Read the model definition and answer for the solid it produces. Units are mm, in the model's axes. A direction names the side the tool comes from. Give positions to 0.01 mm unless a question says otherwise; leave off trailing zeros. Write each loop counter-clockwise with the first axis right and the second up, starting at its lowest first coordinate (ties: lowest second). Pieces come first, ordered by that corner, then holes. Notation, with made-up numbers: M -18,-16 L 24,-16 A19 cw 24,1 Z; hole C 87.5,16.25 d7. An arc over 180 degrees is marked long. Put each result on its own line as item: value.
from build123d import *

# Parameters (mm, degrees)
SKETCH1_R                 = 4.7625
SKETCH1_W                 = 6.5278
SKETCH1_H                 = 6.5278
SKETCH1_H_2               = 6.348837221
BOSS_EXTRUDE1_DEPTH       = 6.35
F_6_CLEARANCE_HOLE1_D     = 3.7973
F_6_CLEARANCE_HOLE1_DEPTH = 12.7
F_6_CLEARANCE_HOLE1_TIP   = 1.140824014
SKETCH7_W                 = 6.35
SKETCH7_H                 = 6.1722
BOSS_EXTRUDE2_DEPTH       = 1.016
SKETCH8_W                 = 6.35
SKETCH8_H                 = 6.1722
BOSS_EXTRUDE3_DEPTH       = 1.016
SKETCH9_R                 = 1.5875
CUT_EXTRUDE1_DEPTH        = 161.894515133


with BuildPart() as part:
    # Sketch1 → Boss-Extrude1 (new body)
    with BuildSketch(Plane(origin=(0, 0, 0), x_dir=(0, 0, -1), z_dir=(1, 0, 0))):
        Polygon((0, 0), (-14.664696837, 25.4), (-144.085303163, 25.4), (-158.75, 0), align=None)
        with Locations((-130.048, 12.7)):
            Circle(SKETCH1_R, mode=Mode.SUBTRACT)
        with Locations((-28.702, 12.7)):
            Circle(SKETCH1_R, mode=Mode.SUBTRACT)
        with Locations((-17.750796837, 12.6111)):
            Rectangle(SKETCH1_W, SKETCH1_H, mode=Mode.SUBTRACT)
        with Locations((-140.999203163, 12.70058139)):
            Rectangle(SKETCH1_W, SKETCH1_H_2, mode=Mode.SUBTRACT)
        with Locations((-79.4639, 12.7889)):
            Rectangle(SKETCH1_W, SKETCH1_H, mode=Mode.SUBTRACT)
    extrude(amount=BOSS_EXTRUDE1_DEPTH)

    # #6 Clearance Hole1
    with Locations(Plane(origin=(0, 25.4, 0), x_dir=(1, 0, 0), z_dir=(0, 1, 0))):
        with Locations((3.175, -79.375)):
            Hole(F_6_CLEARANCE_HOLE1_D / 2, depth=F_6_CLEARANCE_HOLE1_DEPTH)
            with Locations((0, 0, -(F_6_CLEARANCE_HOLE1_DEPTH + F_6_CLEARANCE_HOLE1_TIP / 2))):  # 118° drill point
                Cone(0, F_6_CLEARANCE_HOLE1_D / 2, F_6_CLEARANCE_HOLE1_TIP, mode=Mode.SUBTRACT)

    # Sketch7 → Boss-Extrude2 (add)
    with BuildSketch(Plane(origin=(0, 0, 0), x_dir=(-1, 0, 0), z_dir=(0, 0.499999999999998, -0.8660254037844397))):
        with Locations((-3.175, 19.893293675)):
            Rectangle(SKETCH7_W, SKETCH7_H)
    extrude(amount=BOSS_EXTRUDE2_DEPTH)

    # Sketch8 → Boss-Extrude3 (add)
    with BuildSketch(Plane(origin=(0, 68.740766425, 119.0625), x_dir=(1, 0, 0), z_dir=(0, 0.500000000000004, 0.8660254037844365))):
        with Locations((3.175, -59.481706325)):
            Rectangle(SKETCH8_W, SKETCH8_H)
    extrude(amount=BOSS_EXTRUDE3_DEPTH)

    # Sketch9 → Cut-Extrude1 (cut, through all)
    with BuildSketch(Plane(origin=(6.35, 0, 0), x_dir=(0, 0, -1), z_dir=(1, 0, 0))):
        with Locations((-151.13, 3.81)):
            Circle(SKETCH9_R)
        with Locations((-7.62, 3.81)):
            Circle(SKETCH9_R)
    extrude(amount=-CUT_EXTRUDE1_DEPTH, mode=Mode.SUBTRACT)


solid = part.part
(1) Given pin 1 Ø1.5 at (x, y) = (5, 2.5) entering from +Z; pin 2 Ø1.9 at (x, y) = (2, 13) entering from -Z; pin 3 Ø2.5 at (x, z) = (3.175, 79.375) entering from +Y (3 decimals); pin 4 Ø7.5 at (y, z) = (12.7, 130.048) entering from -X, each flat-ended and moving along its own axis, determine where each tip first touches the part or whether it passes through.
Result:
pin 1: stops at z = 157.74
pin 2: stops at z = 6.96
pin 3: stops at y = 9.525
pin 4: passes through
(2) Section C-C on x = 4 is taken. Give the number of separate pieces and of enclosed holes in the cut face, and give its area (3 significant figures).
Result:
separate pieces: 1
enclosed holes: 6
area: 3,360 mm²
(3) Straight lines are drawn through the part: line 1 along Y through (x, z) = (2, 19) (3 decimals); line 2 along Z through (x, y) = (4.75, 9.25); line 3 along Z through (x, y) = (1.25, 11.75). For each, find the intervals that lie inside material, in ascending order. Write a range as from..to.
Result:
line 1: y = 0..9.347, 15.875..25.4
line 2: z = 5.34..25.42, 31.99..126.76, 133.33..153.41
line 3: z = 6.78..14.49, 21.01..24.04, 33.37..76.2, 82.73..125.38, 134.71..137.74, 144.26..151.97
(4) Section A-A on z = 17.5 is taken. Determine the outline of the cut face in (x, y) (3 decimals), and give its area (3 significant figures).
Result:
outline: M 0,0 L 6.35,0 L 6.35,9.347 L 0,9.347 Z; M 0,15.875 L 6.35,15.875 L 6.35,25.4 L 0,25.4 Z
area: 120 mm²
(5) For a pull along Y with two mould halves and no side action, classify faces 1 (the face through (5, 25.4, 78)), 2 (the face through (0, 7, 80)), 3 (the face through (3, 13, 21.015)) as +Y half, -Y half, draft (parallel to the pull), parting line (faces both ways), or undercut.
Result:
face 1: +Y half
face 2: draft
face 3: undercut
(6) Section B-B on y = 12.7 is taken. Determine the outline of the cut face in (x, z).
Result:
outline: M 0,7.33 L 6.35,7.33 L 6.35,14.49 L 0,14.49 Z; M 0,21.01 L 6.35,21.01 L 6.35,23.94 L 0,23.94 Z; M 0,33.46 L 6.35,33.46 L 6.35,76.2 L 0,76.2 Z; M 0,82.73 L 6.35,82.73 L 6.35,125.29 L 0,125.29 Z; M 0,134.81 L 6.35,134.81 L 6.35,137.74 L 0,137.74 Z; M 0,144.26 L 6.35,144.26 L 6.35,151.42 L 0,151.42 Z
(7) Which of the six approach directions +Z, -Z, +X, -X, +Y, -Y give full straight-line access (tool end or side, diameter ignored) to faces 4 (the face through (3, 15.875, 141)), 5 (the face through (3.219, 17.774, 9.088))?
Result:
face 4: +X, -X
face 5: -Z, +X, -X, +Y
